Here's how the part is built. I have some questions about the finished solid (model axes, mm). Round coordinates to 2 decimals unless told otherwise and drop trailing zeros. One line per item, written item: value. Start each with the question number.
Item 1: Imagine slicing it at A-A, the plane z = 2.45. Count the separate pieces of the cut face and the enclosed holes in it, then the cut area to 3 significant figures.
Item 2: For P1, Ø1.7, axis at y = 135, z = 0.5, coming from the -X side; P2, Ø1, axis at y = 110, z = 2, coming from the -X side, each with a flat end and sliding along its axis, tell me the tip position at first contact or that it passes through.
Item 3: Thinking about a two-plate mould opening in X: for faces 1 (the face through (-136.67, 28.94, 1.57)), 2 (the face through (-7.559, -5.796, 1.61)), 3 (the face through (15, 15, 0)), 4 (the face through (171.003, 54.52, 1.61)), which applies, released by +X, released by -X, zero draft, split by the parting line, or undercut?
Item 4: If I drill on line 1 (X direction, y = 176.5, z = 2.35); line 2 (Y direction, x = 0, z = 0.8) (3 decimals); line 3 (Y direction, x = -57.5, z = 2.35) (3 decimals), over which ranges is the centre line in solid material (lowest first)?
```python
from build123d import *

# Parameters (mm, degrees)
BOSS_EXTRUDE1_DEPTH = 3.175
CUT_EXTRUDE3_DEPTH  = 1.5875
SKETCH3_R           = 9.525
CUT_EXTRUDE4_DEPTH  = 4.175
CUT_EXTRUDE5_DEPTH  = 4.175
SKETCH8_R           = 2.413
CUT_EXTRUDE7_DEPTH  = 4.175
SKETCH9_R           = 2.413
CUT_EXTRUDE8_DEPTH  = 4.175
FILLET1_R           = 12.7
CUT_EXTRUDE9_DEPTH  = 4.175
FILLET2_R           = 25.4
SKETCH11_R          = 2.2479
CUT_EXTRUDE10_DEPTH = 4.175
SKETCH14_R          = 3.175
BOSS_EXTRUDE2_DEPTH = 3.175
FILLET3_R           = 12.7
FILLET4_R           = 6.35


with BuildPart() as part:
    # Sketch1 → Boss-Extrude1 (new body)
    with BuildSketch(Plane.XY):
        with BuildLine():
            Line((0, 139.7), (139.7, 139.7))
            Line((139.7, 139.7), (174.625, 139.7))
            Line((174.625, 139.7), (174.625, 50.700684167))
            Line((174.625, 50.700684167), (130.175, 50.700684167))
            ThreePointArc((130.175, 50.700684167), (-78.845432404, -115.323405209), (0, 139.7))
        make_face()
    extrude(amount=BOSS_EXTRUDE1_DEPTH)

    # Sketch2 → Cut-Extrude3 (cut)
    with BuildSketch(Plane(origin=(0, 0, 0), x_dir=(-1, 0, 0), z_dir=(0, 0, -1))):
        Polygon((-1.5875, -1.011349039), (-1.5875, -2.491875854), (0, -1.751612446), align=None)
        Polygon((-1.5875, -1.011349039), (0, -1.751612446), (1.5875, -1.011349039), (1.5875, 1.011349039), (0, 1.751612446), (-1.5875, 1.011349039), align=None)
        Polygon((1.5875, -1.011349039), (0, -1.751612446), (1.5875, -2.491875854), align=None)
        Polygon((-3.756345013, 0), (-1.5875, -1.011349039), (-1.5875, 1.011349039), align=None)
        Polygon((-1.5875, 2.491875854), (-1.5875, 1.011349039), (0, 1.751612446), align=None)
        Polygon((0, 1.751612446), (1.5875, 1.011349039), (1.5875, 2.491875854), align=None)
        Polygon((1.5875, 1.011349039), (1.5875, -1.011349039), (3.756345013, 0), align=None)
        with BuildLine():
            ThreePointArc((-127.273929282, -57.597195461), (-126.611197849, -59.039771165), (-125.932116301, -60.474722685))
            Line((-125.932116301, -60.474722685), (-120.185236911, -57.794908815))
            Line((-120.185236911, -57.794908815), (-121.527049892, -54.917381591))
            Line((-121.527049892, -54.917381591), (-127.273929282, -57.597195461))
        make_face()
        with BuildLine():
            Line((121.527049892, 54.917381591), (127.273929282, 57.597195461))
            ThreePointArc((127.273929282, 57.597195461), (126.611197849, 59.039771165), (125.932116301, 60.474722685))
            Line((125.932116301, 60.474722685), (120.185236911, 57.794908815))
            Line((120.185236911, 57.794908815), (121.527049892, 54.917381591))
        make_face()
        with BuildLine():
            Line((120.185236911, -57.794908815), (125.932116301, -60.474722685))
            ThreePointArc((125.932116301, -60.474722685), (126.611197849, -59.039771165), (127.273929282, -57.597195461))
            Line((127.273929282, -57.597195461), (121.527049892, -54.917381591))
            Line((121.527049892, -54.917381591), (120.185236911, -57.794908815))
        make_face()
        with BuildLine():
            Line((0, 139.7), (-1.5875, 139.7))
            Line((-1.5875, 139.7), (-1.5875, 133.35))
            Line((-1.5875, 133.35), (1.5875, 133.35))
            Line((1.5875, 133.35), (1.5875, 139.690979822))
            ThreePointArc((1.5875, 139.690979822), (0.793762813, 139.697744937), (0, 139.7))
        make_face()
    extrude(amount=-CUT_EXTRUDE3_DEPTH, mode=Mode.SUBTRACT)

    # Sketch3 → Cut-Extrude4 (cut, through all)
    with BuildSketch(Plane.XY.offset(3.175)):
        Circle(SKETCH3_R)
    extrude(amount=-CUT_EXTRUDE4_DEPTH, mode=Mode.SUBTRACT)

    # Sketch2_4 → Cut-Extrude5 (cut, through all)
    with BuildSketch(Plane(origin=(0, 0, 0), x_dir=(-1, 0, 0), z_dir=(0, 0, -1))):
        with BuildLine():
            Line((-60.312918166, 26.37276318), (-55.328894815, 24.048674923))
            ThreePointArc((-55.328894815, 24.048674923), (-54.333740605, 25.183430817), (-53.975, 26.649482664))
            ThreePointArc((-53.975, 26.649482664), (-53.978021896, 26.787974218), (-53.987081834, 26.926202147))
            Line((-53.987081834, 26.926202147), (-58.971105185, 29.250290404))
            ThreePointArc((-58.971105185, 29.250290404), (-60.027527224, 27.991295645), (-60.312918166, 26.37276318))
        make_face()
        with BuildLine():
            ThreePointArc((-60.312918166, 26.37276318), (-58.491812981, 23.77195544), (-55.328894815, 24.048674923))
            Line((-55.328894815, 24.048674923), (-60.312918166, 26.37276318))
        make_face()
        with BuildLine():
            Line((-58.971105185, 29.250290404), (-53.987081834, 26.926202147))
            ThreePointArc((-53.987081834, 26.926202147), (-55.808187019, 29.527009887), (-58.971105185, 29.250290404))
        make_face()
        with BuildLine():
            ThreePointArc((53.987081834, 26.926202147), (54.272472776, 25.307669683), (55.328894815, 24.048674923))
            Line((55.328894815, 24.048674923), (60.312918166, 26.37276318))
            ThreePointArc((60.312918166, 26.37276318), (60.321978104, 26.510991109), (60.325, 26.649482664))
            ThreePointArc((60.325, 26.649482664), (59.966259395, 28.115534511), (58.971105185, 29.250290404))
            Line((58.971105185, 29.250290404), (53.987081834, 26.926202147))
        make_face()
        with BuildLine():
            ThreePointArc((58.971105185, 29.250290404), (55.808187019, 29.527009887), (53.987081834, 26.926202147))
            Line((53.987081834, 26.926202147), (58.971105185, 29.250290404))
        make_face()
        with BuildLine():
            Line((60.312918166, 26.37276318), (55.328894815, 24.048674923))
            ThreePointArc((55.328894815, 24.048674923), (58.491812981, 23.77195544), (60.312918166, 26.37276318))
        make_face()
        with BuildLine():
            ThreePointArc((-1.5875, -69.587590332), (-3.175, -72.337220989), (-1.5875, -75.086851646))
            Line((-1.5875, -75.086851646), (-1.5875, -69.587590332))
        make_face()
        with BuildLine():
            Line((-1.5875, -69.587590332), (-1.5875, -75.086851646))
            ThreePointArc((-1.5875, -75.086851646), (0, -75.512220989), (1.5875, -75.086851646))
            Line((1.5875, -75.086851646), (1.5875, -69.587590332))
            ThreePointArc((1.5875, -69.587590332), (0, -69.162220989), (-1.5875, -69.587590332))
        make_face()
        with BuildLine():
            Line((1.5875, -69.587590332), (1.5875, -75.086851646))
            ThreePointArc((1.5875, -75.086851646), (2.749630657, -73.924720989), (3.175, -72.337220989))
            ThreePointArc((3.175, -72.337220989), (2.749630657, -70.749720989), (1.5875, -69.587590332))
        make_face()
    extrude(amount=-CUT_EXTRUDE5_DEPTH, mode=Mode.SUBTRACT)

    # Sketch8 → Cut-Extrude7 (cut, through all)
    with BuildSketch(Plane.XY.offset(3.175)):
        with Locations((25.0825, 101.6)):
            Circle(SKETCH8_R)
        with Locations((-25.0825, 101.6)):
            Circle(SKETCH8_R)
        with Locations((-25.0825, 127)):
            Circle(SKETCH8_R)
        with Locations((25.0825, 127)):
            Circle(SKETCH8_R)
        with Locations((102.681193713, -20.205550325)):
            Circle(SKETCH8_R)
        with Locations((125.701411504, -30.940054173)):
            Circle(SKETCH8_R)
        with Locations((81.480548613, -65.670480461)):
            Circle(SKETCH8_R)
        with Locations((104.500766404, -76.404984309)):
            Circle(SKETCH8_R)
        with Locations((-81.480548613, -65.670480461)):
            Circle(SKETCH8_R)
        with Locations((-104.500766404, -76.404984309)):
            Circle(SKETCH8_R)
        with Locations((-102.681193713, -20.205550325)):
            Circle(SKETCH8_R)
        with Locations((-125.701411504, -30.940054173)):
            Circle(SKETCH8_R)
    extrude(amount=-CUT_EXTRUDE7_DEPTH, mode=Mode.SUBTRACT)

    # Sketch9 → Cut-Extrude8 (cut, through all)
    with BuildSketch(Plane.XY.offset(3.175)):
        with Locations((100.6475, 123.825)):
            Circle(SKETCH9_R)
        with Locations((63.8175, 123.825)):
            Circle(SKETCH9_R)
        with Locations((63.8175, 104.775)):
            Circle(SKETCH9_R)
        with Locations((100.6475, 104.775)):
            Circle(SKETCH9_R)
        with BuildLine():
            Line((99.06, 121.412), (100.6475, 121.412))
            ThreePointArc((100.6475, 121.412), (98.2345, 123.825000007), (100.647500013, 126.238))
            Line((100.647500013, 126.238), (99.06, 126.238))
            ThreePointArc((99.06, 126.238), (96.647, 123.825), (99.06, 121.412))
        make_face()
        with BuildLine():
            Line((100.6475, 121.412), (102.235, 121.412))
            ThreePointArc((102.235, 121.412), (104.648, 123.825), (102.235, 126.238))
            Line((102.235, 126.238), (100.647500013, 126.238))
            ThreePointArc((100.647500013, 126.238), (102.353748668, 125.531248658), (103.0605, 123.825))
            ThreePointArc((103.0605, 123.825), (102.353748663, 122.118751337), (100.6475, 121.412))
        make_face()
        with BuildLine():
            ThreePointArc((100.6475, 102.362), (98.2345, 104.775), (100.6475, 107.188))
            Line((100.6475, 107.188), (99.06, 107.188))
            ThreePointArc((99.06, 107.188), (96.647, 104.775), (99.06, 102.362))
            Line((99.06, 102.362), (100.6475, 102.362))
        make_face()
        with BuildLine():
            ThreePointArc((102.235, 102.362), (104.648, 104.775), (102.235, 107.188))
            Line((102.235, 107.188), (100.6475, 107.188))
            ThreePointArc((100.6475, 107.188), (102.353748663, 106.481248663), (103.0605, 104.775))
            ThreePointArc((103.0605, 104.775), (102.353748663, 103.068751337), (100.6475, 102.362))
            Line((100.6475, 102.362), (102.235, 102.362))
        make_face()
    extrude(amount=-CUT_EXTRUDE8_DEPTH, mode=Mode.SUBTRACT)

    # Fillet1
    fillet1_edges = [part.edges().sort_by_distance(p)[0] for p in [
        (174.625, 139.7, 1.5875),
        (174.625, 50.700684167, 1.5875),
        (130.175, 50.700684167, 1.5875),
    ]]
    fillet(fillet1_edges, radius=FILLET1_R)

    # Sketch10 → Cut-Extrude9 (cut, through all)
    with BuildSketch(Plane.XY.offset(3.175)):
        with BuildLine():
            Line((87.894185103, -108.585), (-87.894185103, -108.585))
            ThreePointArc((-87.894185103, -108.585), (0, -139.7), (87.894185103, -108.585))
        make_face()
    extrude(amount=-CUT_EXTRUDE9_DEPTH, mode=Mode.SUBTRACT)

    # Fillet2
    fillet2_edges = [part.edges().sort_by_distance(p)[0] for p in [
        (-87.894185103, -108.585, 1.5875),
        (87.894185103, -108.585, 1.5875),
    ]]
    fillet(fillet2_edges, radius=FILLET2_R)

    # Sketch11 → Cut-Extrude10 (cut, through all)
    with BuildSketch(Plane.XY.offset(3.175)):
        with Locations((-93.58045976, 10.312378308)):
            Circle(SKETCH11_R)
        with Locations((-105.090568655, 4.945126384)):
            Circle(SKETCH11_R)
        with Locations((-52.252619944, -78.315460186)):
            Circle(SKETCH11_R)
        with Locations((-63.76272884, -83.68271211)):
            Circle(SKETCH11_R)
        with Locations((52.252619944, -78.315460186)):
            Circle(SKETCH11_R)
        with Locations((63.76272884, -83.68271211)):
            Circle(SKETCH11_R)
        with Locations((-48.895, 93.1545)):
            Circle(SKETCH11_R)
        with Locations((-48.895, 80.4545)):
            Circle(SKETCH11_R)
    extrude(amount=-CUT_EXTRUDE10_DEPTH, mode=Mode.SUBTRACT)

    # Sketch14 → Boss-Extrude2 (add)
    with BuildSketch(Plane(origin=(0, 0, 0), x_dir=(-1, 0, 0), z_dir=(0, 0, -1))):
        with BuildLine():
            Line((-38.1, 139.7), (-38.1, 202.565))
            Line((-38.1, 202.565), (38.1, 202.565))
            Line((38.1, 202.565), (38.1, 134.404166602))
            ThreePointArc((38.1, 134.404166602), (19.233147502, 138.369707802), (0, 139.7))
            Line((0, 139.7), (-38.1, 139.7))
        make_face()
        with Locations((-24.257, 177.165)):
            Circle(SKETCH14_R, mode=Mode.SUBTRACT)
        with Locations((24.257, 177.165)):
            Circle(SKETCH14_R, mode=Mode.SUBTRACT)
        with Locations((24.257, 158.115)):
            Circle(SKETCH14_R, mode=Mode.SUBTRACT)
        with Locations((-24.257, 158.115)):
            Circle(SKETCH14_R, mode=Mode.SUBTRACT)
    extrude(amount=-BOSS_EXTRUDE2_DEPTH)

    # Fillet3
    fillet3_edges = [part.edges().sort_by_distance(p)[0] for p in [
        (38.1, 202.565, 1.5875),
        (-38.1, 202.565, 1.5875),
    ]]
    fillet(fillet3_edges, radius=FILLET3_R)

    # Fillet4
    fillet4_edges = [part.edges().sort_by_distance(p)[0] for p in [
        (-38.1, 134.404166602, 1.5875),
        (38.1, 139.7, 1.5875),
    ]]
    fillet(fillet4_edges, radius=FILLET4_R)


solid = part.part
```
Values follow:
1. separate pieces: 1
1. enclosed holes: 32
1. area: 68,500 mm^2
2. P1: stops at x = -40.5
2. P2: stops at x = -86.75
3. face 1: released by -X
3. face 2: undercut
3. face 3: zero draft
3. face 4: released by +X
4. line 1: x = -38.1 to -27.36, -21.15 to 21.15, 27.36 to 38.1
4. line 2: y = -108.585 to -75.512, -69.162 to -9.525, 9.525 to 133.35, 139.7 to 202.565
4. line 3: y = -108.585 to 23.494, 29.805 to 127.318
